Part print with two shaded views. Sizes in mm from the minimum x, y, z corner. A direction names the side the tool comes from. Coordinates: 2 decimals unless noted, no trailing zeros. Loops run counter-clockwise (first coordinate to the right, second up) from the corner with the lowest first, then second, coordinate; pieces in that order, holes last.
(1) Flat gauge pins, fed straight in: P1, Ø3, axis at x = 18.5, y = 3, coming from the -Z side; P2, Ø3, axis at y = 2, z = 17, coming from the +X side; P3, Ø1.5, axis at y = 4, z = 31, coming from the -X side. Where does each tip first touch, or does it go through?
(2) Slice it at A-A (y = 2.55). Give the cut face in (x, z).
(3) Wall check: L1, parallel to X at y = 2.6, z = 28; L2, parallel to X at y = 2, z = 23; L3, parallel to X at y = 3.25, z = 5. Give the ranges that are in metal, low to high.
(4) Slice it at C-C (x = 32). Give the cut face in (y, z), and give its area (3 significant figures).
(5) Slice it at B-B (z = 9). Give the cut face in (x, y), and give its area (3 significant figures).
(6) Tool access for the marked faces 1, 2 and 3: list every direction of +Z, -Z, +X, -X, +Y, -Y with a clear straight run to the whole face (end or side of a thin tool).
(7) Slice it at D-D (z = 30.5). Give the cut face in (x, y), and give its area (3 significant figures).
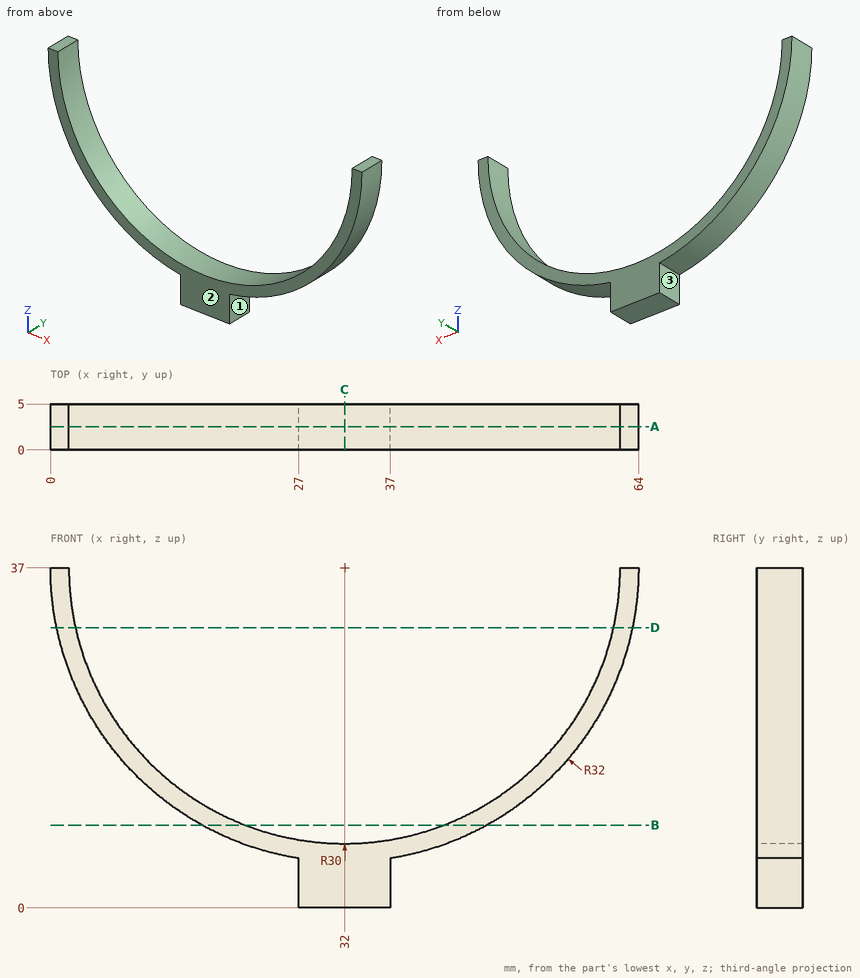
Response values:
1. P1: stops at z = 7.34
1. P2: stops at x = 58.11
1. P3: stops at x = 0.43
2. outline: (0, 37) arc R32 ccw to (27, 5.39) - (27, 0) - (37, 0) - (37, 5.39) arc R32 ccw to (64, 37) - (62, 37) arc R30 cw to (2, 37) - close
3. L1: x = 1.29 to 3.38, 60.62 to 62.71
3. L2: x = 3.23 to 5.47, 58.53 to 60.77
3. L3: x = 27 to 37
4. outline: (0, 0) - (5, 0) - (5, 7) - (0, 7) - close
4. area: 35.0 mm2
5. outline: (16.51, 0) - (21.23, 0) - (21.23, 5) - (16.51, 5) - close; (42.77, 0) - (47.49, 0) - (47.49, 5) - (42.77, 5) - close
5. area: 47.2 mm2
6. face 1: -Z, +X, +Y, -Y
6. face 2: +Z, -Z, +X, -X, -Y
6. face 3: -Z, -X, +Y, -Y
7. outline: (0.67, 0) - (2.71, 0) - (2.71, 5) - (0.67, 5) - close; (61.29, 0) - (63.33, 0) - (63.33, 5) - (61.29, 5) - close
7. area: 20.5 mm2
